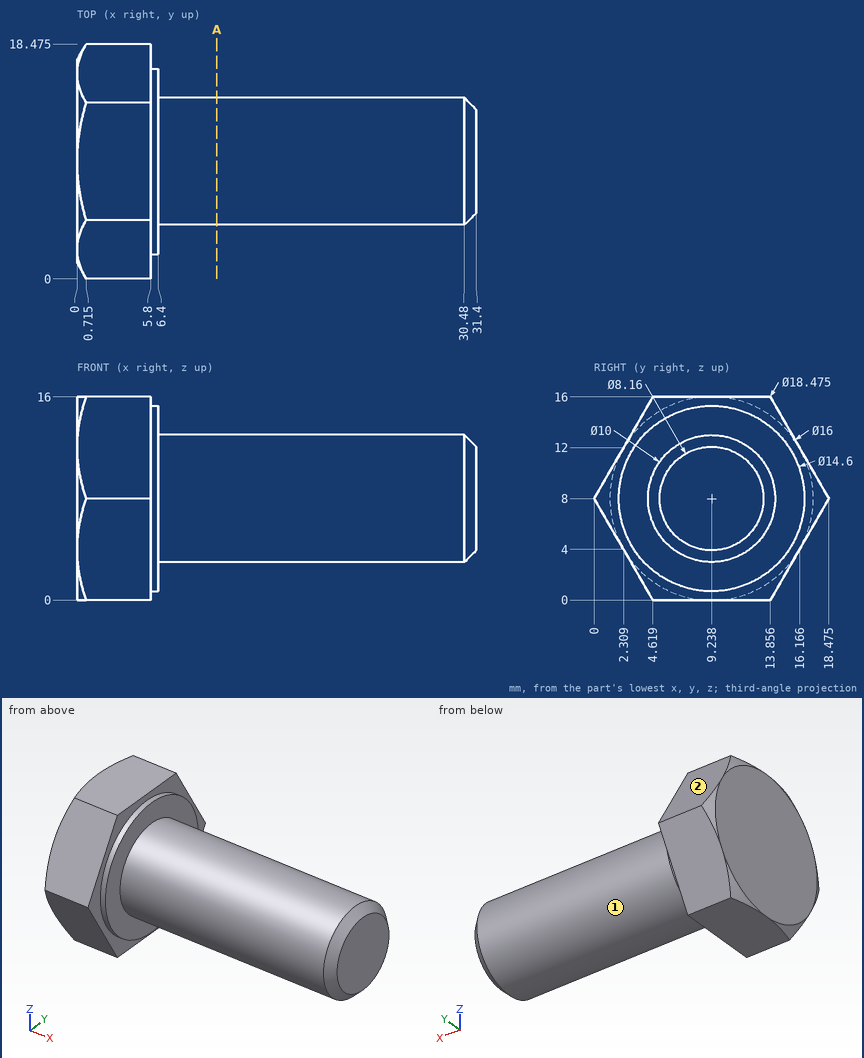
Input: dimensioned drawing with shaded views. Units: mm. Origin: part minimum x, y, z. A direction names the side the tool comes from. Round coordinates to 2 decimals unless told otherwise and drop trailing zeros. Loops run counter-clockwise (first coordinate to the right, second up) from the corner with the lowest first, then second, coordinate; pieces in that order, holes last. Notation, with made-up numbers: (17, 34.5) -> (69, 34.5) arc R21 ccw to (69, 48.5) -> close; hole circle Ø4 at (58, 11.5). An arc over 180 degrees is marked (long way). Use one line per item in the form item = value. Start each with the question number.
1) Section A-A on x = 11. Output: boundary loops of the cut face in (y, z).
2) Access query for the marked faces 1 and 2. Directions: +Z, -Z, +X, -X, +Y, -Y. A direction counts if a zero-diameter tool reaches every point of the face in a straight line with its end or side. Return the directions, or none.
3) First-contact query: P1, Ø8, axis at y = 16.5, z = 13.5, coming from the +X side; P2, Ø4, axis at x = 14, z = 2.5, coming from the -Y side (1 decimal); P3, Ø1, axis at x = 13, y = 9.5, coming from the -Z side. Flat tips, straight axial feed; report the tip coordinate or a pass-through.
4) Line query: L1, parallel to X at y = 2.75, z = 5; L2, parallel to Z at x = 27, y = 9.5; L3, parallel to X at y = 2, z = 6.75. Output: solid intervals per line, ascending.
Response:
q1.outline = circle Ø10 at (9.24, 8)
q2.face_1 = +X
q2.face_2 = +Z, +X, -X, +Y
q3.P1 = 6.4
q3.P2 = 5.7
q3.P3 = 3
q4.L1 = 0 to 6.4
q4.L2 = 3.01 to 12.99
q4.L3 = 0 to 5.8
